Model file for the job. Use its own axes, mm. Round coordinates to 2 decimals unless told otherwise and drop trailing zeros. Order: outer loops, then holes, each group sorted by start corner. A loop starts at its lowest first (then second) coordinate and runs counter-clockwise, first axis right, second up. Notation, with made-up numbers: M -40,-28 L -23,-28 A12 cw -23,-8 Z; hole C 21.5,-38 d1. An arc over 180 degrees is marked long. Return JSON: item names as keys, results as strings. Group by question number.
Item 1: Pin check, flat tips, straight feed: pin 1 Ø0.9 at (y, z) = (1, -229.5) entering from +X; pin 2 Ø1.5 at (x, y) = (30.5, 1) entering from -Z; pin 3 Ø0.5 at (x, y) = (49, 1.5) entering from -Z; pin 4 Ø12 at (x, z) = (27.5, -234.5) entering from -Y. Stop position of each tip, or through.
Item 2: Slice it at A-A on z = -132. Write the cut outline in (x, y), then the cut area to 3 significant figures.
Item 3: Probe line 1 along X through (y, z) = (1, -148); line 2 along X through (y, z) = (0.2, -253); line 3 along Z through (x, y) = (17, 2.7). List the from-to ranges inside material, lowest first.
from build123d import *

# Parameters (mm, degrees)
SALIENTE_EXTRUIR1_DEPTH = 3


with BuildPart() as part:
    # Croquis1 → Saliente-Extruir1 (new body)
    with BuildSketch(Plane(origin=(0, 0, 0), x_dir=(1, 0, 0), z_dir=(0, 1, 0))):
        with BuildLine():
            Line((0, 0), (60, 0))
            Line((60, 0), (60, 210))
            Line((60, 210), (58.8, 210))
            Line((58.8, 210), (58.8, 213))
            Line((58.8, 213), (57.6, 213))
            Line((57.6, 213), (57.6, 216))
            Line((57.6, 216), (56.6, 216))
            Line((56.6, 216), (56.6, 219))
            Line((56.6, 219), (55.6, 219))
            Line((55.6, 219), (55.6, 222))
            Line((55.6, 222), (54.6, 222))
            Line((54.6, 222), (54.6, 225))
            Line((54.6, 225), (53.6, 225))
            Line((53.6, 225), (53.6, 228))
            Line((53.6, 228), (52.6, 228))
            Line((52.6, 228), (52.6, 231))
            Line((52.6, 231), (51.6, 231))
            Line((51.6, 231), (51.6, 234))
            Line((51.6, 234), (50.6, 234))
            Line((50.6, 234), (50.6, 237))
            Line((50.6, 237), (49.6, 237))
            Line((49.6, 237), (49.6, 240))
            Line((49.6, 240), (48.6, 240))
            Line((48.6, 240), (48.6, 243))
            Line((48.6, 243), (47.6, 243))
            Line((47.6, 243), (47.6, 246))
            Line((47.6, 246), (46.6, 246))
            Line((46.6, 246), (46.6, 249))
            Line((46.6, 249), (45.6, 249))
            Line((45.6, 249), (45.6, 252))
            Line((45.6, 252), (44.6, 252))
            Line((44.6, 252), (44.6, 255))
            Line((44.6, 255), (43.6, 255))
            Line((43.6, 255), (43.6, 258))
            Line((43.6, 258), (42.6, 258))
            Line((42.6, 258), (42.6, 261))
            Line((42.6, 261), (41.6, 261))
            Line((41.6, 261), (41.6, 264))
            Line((41.6, 264), (40.575, 264))
            Line((40.575, 264), (40.575, 267))
            ThreePointArc((40.575, 267), (37.990404402, 273.927052945), (31.5, 277.468076471))
            Line((31.5, 277.468076471), (31.5, 115))
            Line((31.5, 115), (28.5, 115))
            Line((28.5, 115), (28.5, 277.468076471))
            ThreePointArc((28.5, 277.468076471), (22.009595598, 273.927052945), (19.425, 267))
            Line((19.425, 267), (19.425, 264))
            Line((19.425, 264), (18.4, 264))
            Line((18.4, 264), (18.4, 261))
            Line((18.4, 261), (17.4, 261))
            Line((17.4, 261), (17.4, 258))
            Line((17.4, 258), (16.4, 258))
            Line((16.4, 258), (16.4, 255))
            Line((16.4, 255), (15.4, 255))
            Line((15.4, 255), (15.4, 252))
            Line((15.4, 252), (14.4, 252))
            Line((14.4, 252), (14.4, 249))
            Line((14.4, 249), (13.4, 249))
            Line((13.4, 249), (13.4, 246))
            Line((13.4, 246), (12.4, 246))
            Line((12.4, 246), (12.4, 243))
            Line((12.4, 243), (11.4, 243))
            Line((11.4, 243), (11.4, 240))
            Line((11.4, 240), (10.4, 240))
            Line((10.4, 240), (10.4, 237))
            Line((10.4, 237), (9.4, 237))
            Line((9.4, 237), (9.4, 234))
            Line((9.4, 234), (8.4, 234))
            Line((8.4, 234), (8.4, 231))
            Line((8.4, 231), (7.4, 231))
            Line((7.4, 231), (7.4, 228))
            Line((7.4, 228), (6.4, 228))
            Line((6.4, 228), (6.4, 225))
            Line((6.4, 225), (5.4, 225))
            Line((5.4, 225), (5.4, 222))
            Line((5.4, 222), (4.4, 222))
            Line((4.4, 222), (4.4, 219))
            Line((4.4, 219), (3.4, 219))
            Line((3.4, 219), (3.4, 216))
            Line((3.4, 216), (2.4, 216))
            Line((2.4, 216), (2.4, 213))
            Line((2.4, 213), (1.2, 213))
            Line((1.2, 213), (1.2, 210))
            Line((1.2, 210), (0, 210))
            Line((0, 210), (0, 0))
        make_face()
    extrude(amount=SALIENTE_EXTRUIR1_DEPTH)


solid = part.part
Output values:
{
 "1": {"pin 1": "x = 52.6", "pin 2": "z = -115", "pin 3": "z = -240", "pin 4": "y = 0"},
 "2": {"outline": "M 0,0 L 28.5,0 L 28.5,3 L 0,3 Z; M 31.5,0 L 60,0 L 60,3 L 31.5,3 Z", "area": "171 mm²"},
 "3": {"line 1": "0 to 28.5, 31.5 to 60", "line 2": "15.4 to 28.5, 31.5 to 44.6", "line 3": "-258 to 0"}
}
